Can you work these out from the model? Positions are in its coordinate system, mm. Face numbers are marked on the shaded views. Give positions to 0.01 mm unless a question says otherwise; leave off trailing zeros. Loops run counter-clockwise (first coordinate to the right, second up) from the corner with the lowest first, then second, coordinate; pieces in that order, holes last. Notation, with made-up numbers: M 30,-3 L 85,-3 A26 cw 85,21 Z; hole C 89,41.5 d7. An arc over 180 degrees is marked long. One line per item, written item: value. Start each with the question number.
from build123d import *
from OCP.BRepFilletAPI import BRepFilletAPI_MakeChamfer

# Parameters (mm, degrees)
BOSS_EXTRUDE1_DEPTH = 12
BOSS_EXTRUDE2_DEPTH = 2
BOSS_EXTRUDE3_DEPTH = 2
FILLET1_R           = 1
CHAMFER2_SIZE       = 5
CHAMFER2_SIZE2      = 1
BOSS_EXTRUDE4_START = -2
SKETCH3_W           = 1.836045909
SKETCH3_H           = 61.241929872
SKETCH3_W_2         = 2.002550415
SKETCH3_H_2         = 60.908326167
BOSS_EXTRUDE4_DEPTH = 2
FILLET2_R           = 2
BOSS_EXTRUDE6_DEPTH = 0.5
CHAMFER3_SIZE       = 3
BOSS_EXTRUDE7_START = -9.956145
BOSS_EXTRUDE7_DEPTH = 9.956145


with BuildPart() as part:
    # Sketch1 → Boss-Extrude1 (new body)
    with BuildSketch(Plane(origin=(0, 0, 0), x_dir=(1, 0, 0), z_dir=(0, 1, 0))):
        with BuildLine():
            Line((-30.01220756, 39.409237307), (16.58779244, 39.409237307))
            ThreePointArc((16.58779244, 39.409237307), (29.315714501, 34.137159368), (34.58779244, 21.409237307))
            Line((34.58779244, 21.409237307), (34.58779244, -25.190762693))
            ThreePointArc((34.58779244, -25.190762693), (29.315714501, -37.918684754), (16.58779244, -43.190762693))
            Line((16.58779244, -43.190762693), (-30.01220756, -43.190762693))
            ThreePointArc((-30.01220756, -43.190762693), (-42.740129621, -37.918684754), (-48.01220756, -25.190762693))
            Line((-48.01220756, -25.190762693), (-48.01220756, 21.409237307))
            ThreePointArc((-48.01220756, 21.409237307), (-42.740129621, 34.137159368), (-30.01220756, 39.409237307))
        make_face()
        with BuildLine():
            ThreePointArc((-31.01220756, 37.409237307), (-41.618809278, 33.015839025), (-46.01220756, 22.409237307))
            Line((-46.01220756, 22.409237307), (-46.01220756, -26.190762693))
            ThreePointArc((-46.01220756, -26.190762693), (-41.618809278, -36.797364411), (-31.01220756, -41.190762693))
            Line((-31.01220756, -41.190762693), (17.58779244, -41.190762693))
            ThreePointArc((17.58779244, -41.190762693), (28.194394158, -36.797364411), (32.58779244, -26.190762693))
            Line((32.58779244, -26.190762693), (32.58779244, 22.409237307))
            ThreePointArc((32.58779244, 22.409237307), (28.194394158, 33.015839025), (17.58779244, 37.409237307))
            Line((17.58779244, 37.409237307), (-31.01220756, 37.409237307))
        make_face(mode=Mode.SUBTRACT)
    extrude(amount=BOSS_EXTRUDE1_DEPTH)

    # Sketch1<3> → Boss-Extrude2 (add)
    with BuildSketch(Plane(origin=(0, 0, 0), x_dir=(1, 0, 0), z_dir=(0, 1, 0))):
        with BuildLine():
            Line((-31.01220756, 37.409237307), (17.58779244, 37.409237307))
            ThreePointArc((17.58779244, 37.409237307), (28.194394158, 33.015839025), (32.58779244, 22.409237307))
            Line((32.58779244, 22.409237307), (32.58779244, -26.190762693))
            ThreePointArc((32.58779244, -26.190762693), (28.194394158, -36.797364411), (17.58779244, -41.190762693))
            Line((17.58779244, -41.190762693), (-31.01220756, -41.190762693))
            ThreePointArc((-31.01220756, -41.190762693), (-41.618809278, -36.797364411), (-46.01220756, -26.190762693))
            Line((-46.01220756, -26.190762693), (-46.01220756, 22.409237307))
            ThreePointArc((-46.01220756, 22.409237307), (-41.618809278, 33.015839025), (-31.01220756, 37.409237307))
        make_face()
        with BuildLine():
            ThreePointArc((-33.01220756, 35.409237307), (-40.790382153, 32.1874119), (-44.01220756, 24.409237307))
            Line((-44.01220756, 24.409237307), (-44.01220756, -28.190762693))
            ThreePointArc((-44.01220756, -28.190762693), (-40.790382153, -35.968937286), (-33.01220756, -39.190762693))
            Line((-33.01220756, -39.190762693), (19.58779244, -39.190762693))
            ThreePointArc((19.58779244, -39.190762693), (27.365967033, -35.968937286), (30.58779244, -28.190762693))
            Line((30.58779244, -28.190762693), (30.58779244, 24.409237307))
            ThreePointArc((30.58779244, 24.409237307), (27.365967033, 32.1874119), (19.58779244, 35.409237307))
            Line((19.58779244, 35.409237307), (-33.01220756, 35.409237307))
        make_face(mode=Mode.SUBTRACT)
    extrude(amount=BOSS_EXTRUDE2_DEPTH)

    # Sketch2 → Boss-Extrude3 (add)
    with BuildSketch(Plane.XZ):
        Polygon((-43.965284719, -28.409237307), (31.645799766, -28.409237307), (28.962058079, -33.229552195), (23.454257131, -35.92314828), (-39.267624427, -35.92314828), (-41.596405872, -34.261761517), align=None)
        Polygon((-43.464319503, 32.190762693), (31.986692978, 32.190762693), (24.084814063, 40.906543889), (12.932368974, 40.906543889), (-33.320922397, 40.906543889), (-40.968109046, 37.811254055), align=None)
    extrude(amount=-BOSS_EXTRUDE3_DEPTH)

    # Fillet1
    fillet1_edges = [part.edges().sort_by_distance(p)[0] for p in [
        (-6.71220756, 2, -37.409237307),
        (32.58779244, 2, 1.890762693),
        (28.194394158, 2, -33.015839025),
        (-41.618809278, 2, -33.015839025),
        (-46.01220756, 2, 1.890762693),
        (-41.618809278, 2, 36.797364411),
        (-6.71220756, 2, 41.190762693),
        (28.194394158, 2, 36.797364411),
    ]]
    fillet(fillet1_edges, radius=FILLET1_R)

    # Chamfer2: one chamfer whose edges measure the first distance from different faces: ONE call of the kernel's chamfer builder (chamfer() names one face for all edges)
    chamfer2_edges_1 = [part.edges().sort_by_distance(p)[0] for p in [
        (-6.71220756, 12, -39.409237307),
    ]]
    chamfer2_side_1 = [part.faces().sort_by_distance(p)[0] for p in [
        (-6.71220756, 6, -39.409237307),
    ]]
    chamfer2_edges_2 = [part.edges().sort_by_distance(p)[0] for p in [
        (-42.740129621, 12, -34.137159368),
    ]]
    chamfer2_side_2 = [part.faces().sort_by_distance(p)[0] for p in [
        (-42.740129621, 6, -34.137159368),
    ]]
    chamfer2_edges_3 = [part.edges().sort_by_distance(p)[0] for p in [
        (-48.01220756, 12, 1.890762693),
    ]]
    chamfer2_side_3 = [part.faces().sort_by_distance(p)[0] for p in [
        (-48.01220756, 6, 1.890762693),
    ]]
    chamfer2_edges_4 = [part.edges().sort_by_distance(p)[0] for p in [
        (-42.740129621, 12, 37.918684754),
    ]]
    chamfer2_side_4 = [part.faces().sort_by_distance(p)[0] for p in [
        (-42.740129621, 6, 37.918684754),
    ]]
    chamfer2_edges_5 = [part.edges().sort_by_distance(p)[0] for p in [
        (-6.71220756, 12, 43.190762693),
    ]]
    chamfer2_side_5 = [part.faces().sort_by_distance(p)[0] for p in [
        (-6.71220756, 6, 43.190762693),
    ]]
    chamfer2_edges_6 = [part.edges().sort_by_distance(p)[0] for p in [
        (29.315714501, 12, 37.918684754),
    ]]
    chamfer2_side_6 = [part.faces().sort_by_distance(p)[0] for p in [
        (29.315714501, 6, 37.918684754),
    ]]
    chamfer2_edges_7 = [part.edges().sort_by_distance(p)[0] for p in [
        (34.58779244, 12, 1.890762693),
    ]]
    chamfer2_side_7 = [part.faces().sort_by_distance(p)[0] for p in [
        (34.58779244, 6, 1.890762693),
    ]]
    chamfer2_edges_8 = [part.edges().sort_by_distance(p)[0] for p in [
        (29.315714501, 12, -34.137159368),
    ]]
    chamfer2_side_8 = [part.faces().sort_by_distance(p)[0] for p in [
        (29.315714501, 6, -34.137159368),
    ]]
    chamfer2 = BRepFilletAPI_MakeChamfer(part.part.solid().wrapped)
    for e in chamfer2_edges_1:
        chamfer2.Add(CHAMFER2_SIZE, CHAMFER2_SIZE2, e.wrapped, chamfer2_side_1[0].wrapped)  # the first distance lies on this face
    for e in chamfer2_edges_2:
        chamfer2.Add(CHAMFER2_SIZE, CHAMFER2_SIZE2, e.wrapped, chamfer2_side_2[0].wrapped)  # the first distance lies on this face
    for e in chamfer2_edges_3:
        chamfer2.Add(CHAMFER2_SIZE, CHAMFER2_SIZE2, e.wrapped, chamfer2_side_3[0].wrapped)  # the first distance lies on this face
    for e in chamfer2_edges_4:
        chamfer2.Add(CHAMFER2_SIZE, CHAMFER2_SIZE2, e.wrapped, chamfer2_side_4[0].wrapped)  # the first distance lies on this face
    for e in chamfer2_edges_5:
        chamfer2.Add(CHAMFER2_SIZE, CHAMFER2_SIZE2, e.wrapped, chamfer2_side_5[0].wrapped)  # the first distance lies on this face
    for e in chamfer2_edges_6:
        chamfer2.Add(CHAMFER2_SIZE, CHAMFER2_SIZE2, e.wrapped, chamfer2_side_6[0].wrapped)  # the first distance lies on this face
    for e in chamfer2_edges_7:
        chamfer2.Add(CHAMFER2_SIZE, CHAMFER2_SIZE2, e.wrapped, chamfer2_side_7[0].wrapped)  # the first distance lies on this face
    for e in chamfer2_edges_8:
        chamfer2.Add(CHAMFER2_SIZE, CHAMFER2_SIZE2, e.wrapped, chamfer2_side_8[0].wrapped)  # the first distance lies on this face
    add(Compound.cast(chamfer2.Shape()), mode=Mode.REPLACE)

    # Sketch3 → Boss-Extrude4 (add)
    with BuildSketch(Plane.XZ.offset(BOSS_EXTRUDE4_START)):
        with Locations((29.686081831, 1.878123924)):
            Rectangle(SKETCH3_W, SKETCH3_H)
        with Locations((-43.113419178, 2.044925776)):
            Rectangle(SKETCH3_W_2, SKETCH3_H_2)
    extrude(amount=BOSS_EXTRUDE4_DEPTH)

    # Fillet2
    fillet2_edges = [part.edges().sort_by_distance(p)[0] for p in [
        (28.768058876, 1, 32.190762693),
        (28.768058876, 1, -28.409237307),
        (-42.11214397, 1, 32.190762693),
        (-42.11214397, 1, -28.409237307),
    ]]
    fillet(fillet2_edges, radius=FILLET2_R)

    # Sketch4 → Boss-Extrude6 (add)
    with BuildSketch(Plane.XZ):
        with BuildLine():
            Line((-30.01220756, -39.409237307), (16.58779244, -39.409237307))
            ThreePointArc((16.58779244, -39.409237307), (29.315714501, -34.137159368), (34.58779244, -21.409237307))
            Line((34.58779244, -21.409237307), (34.58779244, 25.190762693))
            ThreePointArc((34.58779244, 25.190762693), (29.315714501, 37.918684754), (16.58779244, 43.190762693))
            Line((16.58779244, 43.190762693), (-30.01220756, 43.190762693))
            ThreePointArc((-30.01220756, 43.190762693), (-42.740129621, 37.918684754), (-48.01220756, 25.190762693))
            Line((-48.01220756, 25.190762693), (-48.01220756, -21.409237307))
            ThreePointArc((-48.01220756, -21.409237307), (-42.740129621, -34.137159368), (-30.01220756, -39.409237307))
        make_face()
        with BuildLine():
            Line((-40.11214397, -28.409237307), (26.768058876, -28.409237307))
            ThreePointArc((26.768058876, -28.409237307), (28.182272439, -27.823450869), (28.768058876, -26.409237307))
            Line((28.768058876, -26.409237307), (28.768058876, 30.190762693))
            ThreePointArc((28.768058876, 30.190762693), (28.182272439, 31.604976255), (26.768058876, 32.190762693))
            Line((26.768058876, 32.190762693), (-40.11214397, 32.190762693))
            ThreePointArc((-40.11214397, 32.190762693), (-41.526357532, 31.604976255), (-42.11214397, 30.190762693))
            Line((-42.11214397, 30.190762693), (-42.11214397, -26.409237307))
            ThreePointArc((-42.11214397, -26.409237307), (-41.526357532, -27.823450869), (-40.11214397, -28.409237307))
        make_face(mode=Mode.SUBTRACT)
    extrude(amount=BOSS_EXTRUDE6_DEPTH)

    # Chamfer3
    chamfer3_edges = [part.edges().sort_by_distance(p)[0] for p in [
        (-42.740129621, -0.5, -34.137159368),
        (-6.71220756, -0.5, -39.409237307),
        (29.315714501, -0.5, -34.137159368),
        (34.58779244, -0.5, 1.890762693),
        (29.315714501, -0.5, 37.918684754),
        (-6.71220756, -0.5, 43.190762693),
        (-42.740129621, -0.5, 37.918684754),
        (-48.01220756, -0.5, 1.890762693),
    ]]
    chamfer(chamfer3_edges, length=CHAMFER3_SIZE)

    # Sketch5 → Boss-Extrude7 (add)
    with BuildSketch(Plane(origin=(0, 12, 0), x_dir=(1, 0, 0), z_dir=(0, 1, 0)).offset(BOSS_EXTRUDE7_START)):
        with BuildLine():
            Line((17.58779244, 37.409237307), (-31.01220756, 37.409237307))
            ThreePointArc((-31.01220756, 37.409237307), (-41.618809278, 33.015839025), (-46.01220756, 22.409237307))
            Line((-46.01220756, 22.409237307), (-46.01220756, -26.190762693))
            ThreePointArc((-46.01220756, -26.190762693), (-41.618809278, -36.797364411), (-31.01220756, -41.190762693))
            Line((-31.01220756, -41.190762693), (17.58779244, -41.190762693))
            ThreePointArc((17.58779244, -41.190762693), (28.194394158, -36.797364411), (32.58779244, -26.190762693))
            Line((32.58779244, -26.190762693), (32.58779244, 22.409237307))
            ThreePointArc((32.58779244, 22.409237307), (28.194394158, 33.015839025), (17.58779244, 37.409237307))
        make_face()
        with BuildLine():
            Line((-30.51220756, 36.909237307), (17.08779244, 36.909237307))
            ThreePointArc((17.08779244, 36.909237307), (27.694394158, 32.515839025), (32.08779244, 21.909237307))
            Line((32.08779244, 21.909237307), (32.08779244, -25.690762693))
            ThreePointArc((32.08779244, -25.690762693), (27.694394158, -36.297364411), (17.08779244, -40.690762693))
            Line((17.08779244, -40.690762693), (-30.51220756, -40.690762693))
            ThreePointArc((-30.51220756, -40.690762693), (-41.118809278, -36.297364411), (-45.51220756, -25.690762693))
            Line((-45.51220756, -25.690762693), (-45.51220756, 21.909237307))
            ThreePointArc((-45.51220756, 21.909237307), (-41.118809278, 32.515839025), (-30.51220756, 36.909237307))
        make_face(mode=Mode.SUBTRACT)
    extrude(amount=BOSS_EXTRUDE7_DEPTH)


solid = part.part
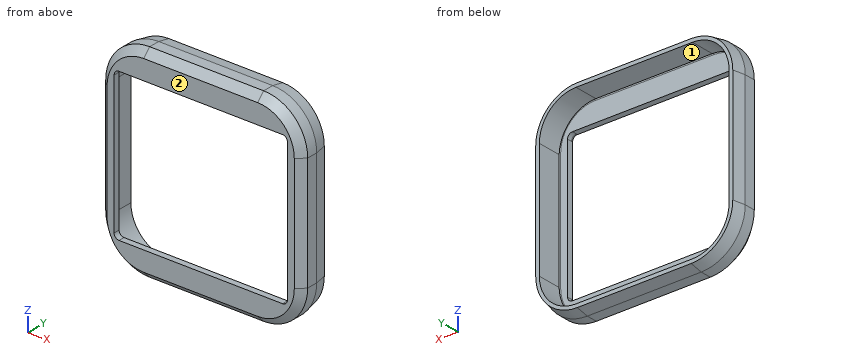
Q1. I need wall thicknesses on line 1 along X through (y, z) = (4, 24.5); line 2 along X through (y, z) = (0, 7); line 3 along Z through (x, y) = (-29, 0). Which ranges of each line are inside material? Lowest first, please.
Q2. If we section it at A-A, the plane y = 4.75: Write out the boundary of the cut face in (x, z).
Q3. For P1, Ø3, axis at y = 6.5, z = 29.5, coming from the +X side; P2, Ø0.8, axis at y = 1.5, z = 11.5, coming from the +X side; P3, Ø1.2, axis at x = 5.5, y = 1.5, coming from the +Z side; P4, Ø1.5, axis at x = -39.5, z = 14.5, coming from the -Y side, each with a flat end and sliding along its axis, tell me the tip position at first contact or that it passes through.
Q4. If we mould it in two halves opening along X, with no side actions, what happens to the marked faces 1 and 2? For each: released by +X, released by -X, zero draft, split by the parting line, or undercut.
Q5. If we section it at C-C, the plane x = -12: Write out the boundary of the cut face in (y, z).
Q6. If we section it at B-B, the plane z = -16.5: Write out the boundary of the cut face in (x, y), plus the area to 3 significant figures.
Q7. If we section it at D-D, the plane y = 9.75: Write out the boundary of the cut face in (x, z), plus the area to 3 significant figures.
Response:
1. line 1: -48.01 to -45.51, 32.09 to 34.59
1. line 2: -45.51 to -42.11, 28.77 to 32.09
1. line 3: -36.91 to -28.41, 32.19 to 40.69
2. outline: M -48.01,-21.41 A18 ccw -30.01,-39.41 L 16.59,-39.41 A18 ccw 34.59,-21.41 L 34.59,25.19 A18 ccw 16.59,43.19 L -30.01,43.19 A18 ccw -48.01,25.19 Z; hole M -45.51,-21.91 A15 ccw -30.51,-36.91 L 17.09,-36.91 A15 ccw 32.09,-21.91 L 32.09,25.69 A15 ccw 17.09,40.69 L -30.51,40.69 A15 ccw -45.51,25.69 Z
3. P1: x = 34.37
3. P2: x = 33.99
3. P3: z = 42.79
3. P4: through
4. face 1: undercut
4. face 2: zero draft
5. outline: M -0.5,-36.41 L 2.5,-39.41 L 7,-39.41 L 12,-38.41 L 12,-36.91 L 2.13,-36.91 A1 cw 2,-36.41 L 2,-28.41 L -0.5,-28.41 Z; M -0.5,32.19 L 2,32.19 L 2,40.19 A1 cw 2.13,40.69 L 12,40.69 L 12,42.19 L 7,43.19 L 2.5,43.19 L -0.5,40.19 Z
6. outline: M -48.01,2.5 L -45.01,-0.5 L -42.11,-0.5 L -42.11,2 L -45.01,2 A1 cw -45.51,2.13 L -45.51,12 L -47.01,12 L -48.01,7 Z; M 28.77,-0.5 L 31.59,-0.5 L 34.59,2.5 L 34.59,7 L 33.59,12 L 32.09,12 L 32.09,2.13 A1 cw 31.59,2 L 28.77,2 Z
6. area: 65.3 mm^2
7. outline: M -47.46,-21.41 A17.45 ccw -30.01,-38.86 L 16.59,-38.86 A17.45 ccw 34.04,-21.41 L 34.04,25.19 A17.45 ccw 16.59,42.64 L -30.01,42.64 A17.45 ccw -47.46,25.19 Z; hole M -45.51,-21.91 A15 ccw -30.51,-36.91 L 17.09,-36.91 A15 ccw 32.09,-21.91 L 32.09,25.69 A15 ccw 17.09,40.69 L -30.51,40.69 A15 ccw -45.51,25.69 Z
7. area: 552 mm^2
